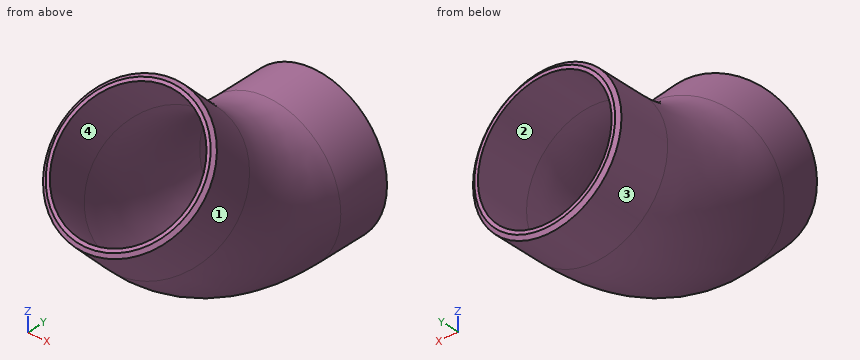
from build123d import *

# Parameters (mm, degrees)
SKETCH2_R    = 16.7005
SKETCH2_R_2  = 15.0495
SCALE1_SCALE = 0.095238095


with BuildPart() as part:
    # Sweep1: sweep along a path in Sketch1
    with BuildLine(Plane(origin=(0, 0, 0), x_dir=(0, 0, -1), z_dir=(1, 0, 0))) as sweep1_path:
        Line((-20.205576272, -20.205576272), (-11.225320151, -11.225320151))
        ThreePointArc((-11.225320151, -11.225320151), (-2.917365657, 1.208412421), (0, 15.875))
        Line((0, 15.875), (0, 28.575))
    # Sketch2 → Sweep1 (sweep)
    with BuildSketch(Plane(origin=(0, 28.575, 0), x_dir=(1, 0, 0), z_dir=(0, 1, 0))):
        Circle(SKETCH2_R)
        Circle(SKETCH2_R_2, mode=Mode.SUBTRACT)
    sweep(path=sweep1_path.line)

    # Sketch3 → Cut-Revolve1 (revolve, cut)
    with BuildSketch(Plane(origin=(0, 0, 0), x_dir=(0, 1, 0), z_dir=(-1, 0, 0))):
        Polygon((27.91720894, 16.7005), (28.575, 16.7005), (28.575, 15.84325), align=None)
    revolve(axis=Axis((0, 28.575, 0), (0, -1, 0)), mode=Mode.SUBTRACT)

    # Sketch3_7 → Cut-Revolve2 (revolve, cut)
    with BuildSketch(Plane(origin=(0, 0, 0), x_dir=(0, 1, 0), z_dir=(-1, 0, 0))):
        Polygon((-31.408445783, -9.002706761), (-32.014613072, -8.396539473), (-31.549484552, -7.931410954), align=None)
    revolve(axis=Axis((0, -11.225320151, 11.225320151), (0, -0.707106781, 0.707106781)), mode=Mode.SUBTRACT)


with BuildPart() as part_1:
    # Scale1: scaled about (0, 1.665203818, 4.020157643)
    add(part.part.scale(SCALE1_SCALE).moved(Location((0, 1.506612978, 3.637285487))))


solid = part_1.part
Source: CAD feature listing. Evaluate the final solid. Frame: model axes, mm. Face numbers are marked on the shaded views. A direction names the side the tool comes from. Give positions to 0.01 mm unless a question says otherwise; leave off trailing zeros. Write each loop counter-clockwise with the first axis right and the second up, starting at its lowest first coordinate (ties: lowest second). Pieces come first, ordered by that corner, then holes. Notation, with made-up numbers: M 87,52.25 L 136,52.25 A14 ccw 136,72.25 Z; hole C -17.5,25 d1. An arc over 180 degrees is marked long. Answer as a JSON object with one key per item and string values.
Q1. Mould query, pull axis Z, two halves, no side actions, for the marked faces 1 and 2. Classes: +Z half, -Z half, draft (parallel to the pull), parting line (faces both ways), or undercut.
Geometry check:
{"face 1": "parting line", "face 2": "undercut"}
Q2. Access query for the marked faces 3 and 4. Directions: +Z, -Z, +X, -X, +Y, -Y. A direction counts if a zero-diameter tool reaches every point of the face in a straight line with its end or side. Return the directions, or none.
Geometry check:
{"face 3": "+Y", "face 4": "none"}
Q3. Cut plane A-A, the plane x = 0. Return the cut outline in (y, z).
Geometry check:
{"outline": "M -1.5,4.39 L -0.69,3.58 A5.24 ccw 3.02,2.05 L 4.17,2.05 L 4.23,2.13 L 4.23,2.2 L 3.02,2.2 A5.08 cw -0.58,3.69 L -1.43,4.55 L -1.48,4.49 Z; M 0.6,6.58 L 1.45,5.72 A2.22 ccw 3.02,5.07 L 4.23,5.07 L 4.23,5.15 L 4.17,5.23 L 3.02,5.23 A2.06 cw 1.56,5.83 L 0.75,6.64 L 0.65,6.63 Z"}
Q4. Ray query, line 1 along Z through (x, y) = (0, 3.5); line 2 along X through (y, z) = (3.95, 4.65); line 3 along Z through (x, y) = (-0.05, 2.5). Return the intervals inside material, ascending.
Geometry check:
{"line 1": "z = 2.05 to 2.2, 5.07 to 5.23", "line 2": "x = -1.23 to -1.01, 1.01 to 1.23", "line 3": "z = 2.07 to 2.23, 5.13 to 5.29"}
Q5. Contact query for flat-ended pins moving along their axis: P1, Ø1.5, axis at x = 1, z = 3.5, coming from the +Y side; P2, Ø1, axis at x = -0.5, z = 3, coming from the -Y side. Output: stop coordinate, or through.
Geometry check:
{"P1": "stops at y = 4.23", "P2": "stops at y = -0.52"}
